Verification items for the finished model (mm, model axes). A direction names the side the tool comes from. Coordinates: 2 decimals unless noted, no trailing zeros. Write each loop counter-clockwise with the first axis right and the second up, starting at its lowest first coordinate (ties: lowest second). Pieces come first, ordered by that corner, then holes. Notation, with made-up numbers: (19.5, -29.5) -> (57.5, -29.5) arc R20 ccw to (57.5, -15.5) -> close; hole circle Ø6 at (22, 72.5). An arc over 180 degrees is marked (long way). Write item = value, one per line. Start each with the question number.
(1) Section check A-A (y = 0). Record the cut outline in (x, z), plus the area to 3 significant figures.
(2) Section check D-D (x = 24). Record the cut outline in (y, z).
(3) Gauge pin test, flat ends, axial feed: pin 1 Ø1 at (x, y) = (21, -1) entering from +Z (3 decimals); pin 2 Ø1.5 at (x, z) = (13, 2) entering from -Y; pin 3 Ø1 at (x, z) = (28, 2) entering from -Y; pin 4 Ø1.8 at (x, y) = (3, -0.01) entering from -Z. Record the tip position at first contact, or that the pin passes through.
(4) Section check B-B (x = 3.5). Record the cut outline in (y, z), plus the area to 3 significant figures.
(5) Set-up check for faces 1 (the face through (4, 0, -2)), 2 (the face through (6, 0, -0.25)): record each of +Z, -Z, +X, -X, +Y, -Y from which the full face is reachable in a straight line by a thin tool's end or side.
(6) Mould release check, pull along Z, two halves, no side actions. Record for faces 3 (the face through (0, 0, -1)), 4 (the face through (6, 0, 0.25)), 5 (the face through (31, 0, 0)), 6 (the face through (18.73, 0.84, -2.67)): released by +Z, released by -Z, zero draft, split by the parting line, or undercut.
(7) Material ranges on probe 1 along X at (y, z) = (-0.4, -1.6); probe 2 along X at (y, z) = (0.15, -1.6); probe 3 along Y at (x, z) = (35, 0.15), recorded low to high. Write a range as [from, to].
(8) Section check C-C (x = 35). Record the cut outline in (y, z).
```python
from build123d import *

# Parameters (mm, degrees)
SKETCH_1_R               = 2.8
EXTRUDE_1_DEPTH          = 38
SKETCH_2_W               = 0.5
SKETCH_2_H               = 5.450532248
CUT_EXTRUDE_1_DEPTH      = 12
CUT_EXTRUDE_2_DEPTH      = 10
CUT_EXTRUDE_2_DEPTH_BACK = 10
SKETCH_3_R               = 1
CUT_EXTRUDE_3_DEPTH      = 10
CUT_EXTRUDE_3_DEPTH_BACK = 10
SKETCH_7_R               = 1


with BuildPart() as part:
    # Sketch 1 → Extrude 1 (new body)
    with BuildSketch(Plane(origin=(0, 0, 0), x_dir=(0, 0, -1), z_dir=(1, 0, 0))):
        Circle(SKETCH_1_R)
    extrude(amount=EXTRUDE_1_DEPTH)

    # Sketch 2 → Cut-Extrude 1 (cut)
    with BuildSketch(Plane.ZY):
        with Locations((0, 0.396255312)):
            Rectangle(SKETCH_2_W, SKETCH_2_H)
    extrude(amount=-CUT_EXTRUDE_1_DEPTH, mode=Mode.SUBTRACT)

    # Sketch 3 → Cut-Extrude 2 (cut, two sides: drawn at the far end of the back side and taken through both)
    with BuildSketch(Plane(origin=(0, 0, 0.25), x_dir=(-1, 0, 0), z_dir=(0, 0, -1)).offset(-CUT_EXTRUDE_2_DEPTH_BACK)):
        with Locations(Location((-3, -0.005591523, 0), (0, 0, 270))):
            Circle(SKETCH_3_R)
        with Locations(Location((-35, -0.005591523, 0), (0, 0, 270))):
            Circle(SKETCH_3_R)
    extrude(amount=CUT_EXTRUDE_2_DEPTH + CUT_EXTRUDE_2_DEPTH_BACK, mode=Mode.SUBTRACT)

    # Sketch 7 → Cut-Extrude 3 (cut, two sides: drawn at the far end of the back side and taken through both)
    with BuildSketch(Plane(origin=(0, 0, 0), x_dir=(1, 0, 0), z_dir=(0, 1, 0)).offset(-CUT_EXTRUDE_3_DEPTH_BACK)):
        with Locations(Location((32, 0, 0), (0, 0, 90))):
            Circle(SKETCH_7_R)
    extrude(amount=CUT_EXTRUDE_3_DEPTH + CUT_EXTRUDE_3_DEPTH_BACK, mode=Mode.SUBTRACT)


solid = part.part
```
Response:
q1.outline = (0, -2.8) -> (2, -2.8) -> (2, -0.25) -> (0, -0.25) -> close; (0, 0.25) -> (2, 0.25) -> (2, 2.8) -> (0, 2.8) -> close; (4, -2.8) -> (34, -2.8) -> (34, 2.8) -> (4, 2.8) -> (4, 0.25) -> (12, 0.25) -> (12, -0.25) -> (4, -0.25) -> close; (36, -2.8) -> (38, -2.8) -> (38, 2.8) -> (36, 2.8) -> close; hole circle Ø2 at (32, 0)
q1.area = 182 mm2
q2.outline = circle Ø5.6 at (0, 0)
q3.pin_1 = 2.755
q3.pin_2 = -2.51
q3.pin_3 = -2.36
q3.pin_4 = through
q4.outline = (-2.33, -0.25) -> (-2.33, 0.25) -> (-0.87, 0.25) -> (-0.87, 2.66) arc R2.8 ccw to (-0.87, -2.66) -> (-0.87, -0.25) -> close; (0.86, -2.66) arc R2.8 ccw to (2.79, -0.25) -> (0.86, -0.25) -> close; (0.86, 0.25) -> (2.79, 0.25) arc R2.8 ccw to (0.86, 2.66) -> close
q4.area = 13.4 mm2
q5.face_1 = +Z, -Z
q5.face_2 = -X, +Y
q6.face_3 = zero draft
q6.face_4 = undercut
q6.face_5 = undercut
q6.face_6 = split by the parting line
q7.probe_1 = [0, 2.08], [3.92, 34.08], [35.92, 38]
q7.probe_2 = [0, 2.01], [3.99, 34.01], [35.99, 38]
q7.probe_3 = [-2.8, -1.01], [0.99, 2.8]
q8.outline = (-1.01, -2.61) -> (-1.01, 2.61) arc R2.8 ccw to start; (0.99, -2.62) arc R2.8 ccw to (0.99, 2.62) -> close
